```python
from build123d import *

# Parameters (mm, degrees)
F0_R     = 3.96875
F1_DEPTH = 50.8
F3_DEPTH = 15.875
F6_DEPTH = 25.4
F8_DEPTH = 25.4


with BuildPart() as f1:
    # F0 (on Front) → F1 (new body)
    with BuildSketch(Plane.XZ):
        with BuildLine():
            Line((-139.7, 0), (0, 0))
            Line((0, 0), (0, 7.903855294))
            add(Edge.make_bspline(
                [(-22.225, 19.05), (-19.6667376265, 16.8833683971), (-15.7418485572, 10.4875386248), (-6.5614327707, 9.3293877219), (0, 7.903855294)],
                knots=[0, 0, 0, 0, 0.4401240907, 1, 1, 1, 1], degree=3))
            Line((-22.225, 19.05), (-139.7, 19.05))
            Line((-139.7, 19.05), (-139.7, 0))
        make_face()
        with Locations((-121.2008071616, 7.5636314338)):
            Circle(F0_R, mode=Mode.SUBTRACT)
        with Locations((-39.9241782725, 7.5636314338)):
            Circle(F0_R, mode=Mode.SUBTRACT)
    extrude(amount=F1_DEPTH)

    # F2 (on face) → F3 (cut)
    with BuildSketch(Plane.XY.offset(19.05)):
        with BuildLine():
            Line((-139.7, -26.4440402389), (-137.8610034316, -26.4440402389))
            ThreePointArc((-137.8610034316, -26.4440402389), (-128.7197553381, -25.3974799855), (-137.8621371984, -24.360870613))
            Line((-137.8621371984, -24.360870613), (-139.7, -24.3874061853))
            Line((-139.7, -24.3874061853), (-139.7, -26.4440402389))
        make_face()
    extrude(amount=-F3_DEPTH, mode=Mode.SUBTRACT)

    # F5 (on face) → F6 (cut)
    with BuildSketch(Plane(origin=(0, 0, 0), x_dir=(1, 0, 0), z_dir=(0, 0, -1))):
        Polygon((-21.9825431705, 50.8), (0, 41.4597280324), (0, 50.8), align=None)
    extrude(amount=-F6_DEPTH, mode=Mode.SUBTRACT)

    # F7 (on face) → F8 (cut)
    with BuildSketch(Plane(origin=(0, 0, 0), x_dir=(1, 0, 0), z_dir=(0, 0, -1))):
        Polygon((0, 9.8713636398), (-21.7288583517, 0), (0, 0), align=None)
    extrude(amount=-F8_DEPTH, mode=Mode.SUBTRACT)


solid = f1.part
```
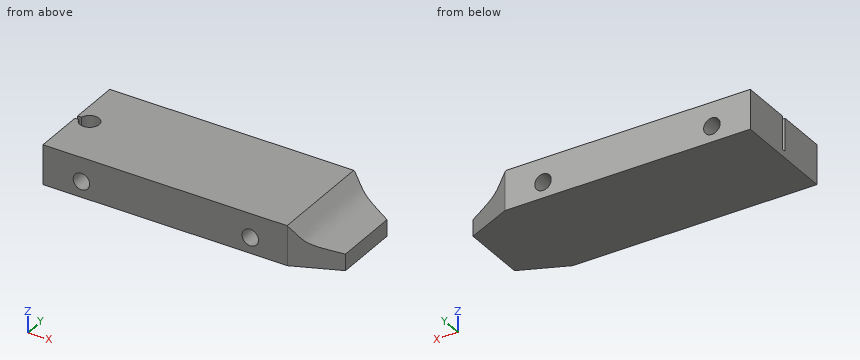
Geometry: final body of the model. Coordinates: model frame, mm. Round coordinates to 2 decimals unless told otherwise and drop trailing zeros. Order: outer loops, then holes, each group sorted by start corner. A loop starts at its lowest first (then second) coordinate and runs counter-clockwise, first axis right, second up. Notation, with made-up numbers: (1.25, -29) - (18.25, -29) arc R29 cw to (18.25, 2) - close; hole circle Ø8 at (-16, -8.5). An arc over 180 degrees is marked (long way). Write item = value, one per line. Start each with the question number.
Q1. Cut plane C-C on y = -46.5. Give the number of separate pieces and of enclosed holes in the cut face, and give its area (3 significant figures).
Q2. Pin query (flat end, axial travel): pin 1 (5 mm diameter, centred on x = -121.2, z = 7.56, fed in from +Y); pin 2 (2 mm diameter, centred on y = -7, z = 7, fed in from +X); pin 3 (5.5 mm diameter, centred on x = -133.35, y = -25.4, fed in from +Z) (3 decimals). Return the tip coordinate at first contact, or that it passes through.
Q3. Ray query, line 1 (Y direction, x = -133.35, z = 6.5); line 2 (X direction, y = -29.5, z = 5.25); line 3 (X direction, y = -7, z = 5.25). Return the intervals inside material, ascending. Write a range as from..to.
Q4. Cut plane B-B on z = 6.25. Return the cut outline in (x, y), and give its area (3 significant figures).
Q5. Cut plane A-A on x = -133.35. Return the cut outline in (y, z) (3 decimals).
Outcome:
q1.separate_pieces = 1
q1.enclosed_holes = 2
q1.area = 2,290 mm^2
q2.pin_1 = through
q2.pin_2 = -4.12
q2.pin_3 = 3.175
q3.line_1 = -50.8..-30.03, -20.77..0
q3.line_2 = -139.7..-135.5, -131.2..-124.43, -117.98..-43.15, -36.7..0
q3.line_3 = -139.7..-124.43, -117.98..-43.15, -36.7..-6.32
q4.outline = (-139.7, -50.8) - (-124.95, -50.8) - (-124.95, 0) - (-139.7, 0) - (-139.7, -24.39) - (-137.86, -24.36) arc R4.63 cw (long way) to (-137.86, -26.44) - (-139.7, -26.44) - close; (-117.46, -50.8) - (-43.67, -50.8) - (-43.67, 0) - (-117.46, 0) - close; (-36.18, -50.8) - (-21.98, -50.8) - (0, -41.46) - (0, -9.87) - (-21.73, 0) - (-36.18, 0) - close
q4.area = 6,050 mm^2
q5.outline = (-50.8, 0) - (0, 0) - (0, 19.05) - (-20.77, 19.05) - (-20.77, 3.175) - (-30.03, 3.175) - (-30.03, 19.05) - (-50.8, 19.05) - close
